Could you check a few things on this model? Use its own coordinates, in mm. Round coordinates to 2 decimals unless told otherwise and drop trailing zeros. Write each loop counter-clockwise with the first axis right and the second up, starting at its lowest first coordinate (ties: lowest second). Pieces come first, ordered by that corner, then holes. Notation, with made-up numbers: M 82,-39.5 L 115,-39.5 A15 ccw 115,-27.5 Z; hole C -25.5,0.5 d4. An arc over 180 degrees is marked long. One line per item, written item: value. Start each with the question number.
(1) I want a section at C-C on x = -9.5. Please give me the cut outline in (y, z).
(2) If I drill on L1, parallel to X at y = -14, z = 1.75; L2, parallel to Y at x = -26, z = 0.5; L3, parallel to X at y = -26, z = 0.5, over which ranges is the centre line in solid material (lowest first)?
(3) I'm going to push a flat-ended pin straight in: pin 1 Ø2.5 at (x, y) = (-36.84, 14.81) entering from +Z. Where does the tip first touch, or does it pass through?
(4) Thinking about a two-plate mould opening in Y: for faces 1 (the face through (39.301, 0, 4)), 2 (the face through (11.99, -24, 3.94)), 3 (the face through (0, -39.298, 4)), which applies, released by +Y, released by -Y, zero draft, split by the parting line, or undercut?
(5) I want a section at B-B on z = 4.75. Count the separate pieces of the cut face and the enclosed holes in it, and give its area (3 significant figures).
(6) I want a section at A-A on x = 7. Please give me the cut outline in (y, z), and give its area (3 significant figures).
```python
from build123d import *

# Parameters (mm, degrees)
SKETCH1_W           = 78.25
SKETCH1_H           = 79.3
SKETCH1_R           = 5
SKETCH1_R_2         = 2
SKETCH1_R_3         = 1.5
BOSS_EXTRUDE1_DEPTH = 8


with BuildPart() as part:
    # Sketch1 → Boss-Extrude1 (new body)
    with BuildSketch(Plane.XY):
        with Locations((0.176122561, 0.352245122)):
            Rectangle(SKETCH1_W, SKETCH1_H)
        with Locations((-9.875194839, -28.39441243)):
            Circle(SKETCH1_R, mode=Mode.SUBTRACT)
        with Locations((9.301122561, -28.217424669)):
            Circle(SKETCH1_R, mode=Mode.SUBTRACT)
        with Locations(Location((-28.948877439, -28.303646558, 0), (0, 0, 180))):
            Circle(SKETCH1_R, mode=Mode.SUBTRACT)
        with Locations((-26.677304512, 19.502245122)):
            Circle(SKETCH1_R_2, mode=Mode.SUBTRACT)
        with Locations((-26.677304512, -8.437754878)):
            Circle(SKETCH1_R_2, mode=Mode.SUBTRACT)
        with Locations((24.122695488, -23.677754878)):
            Circle(SKETCH1_R_2, mode=Mode.SUBTRACT)
        with Locations((25.392695488, 24.582245122)):
            Circle(SKETCH1_R_2, mode=Mode.SUBTRACT)
        with Locations((-36.837723202, 14.814078865)):
            Circle(SKETCH1_R_3, mode=Mode.SUBTRACT)
        with Locations((-36.837723202, -14.185921135)):
            Circle(SKETCH1_R_3, mode=Mode.SUBTRACT)
        with Locations((37.162276798, -14.185921135)):
            Circle(SKETCH1_R_3, mode=Mode.SUBTRACT)
        with Locations((37.162276798, 14.814078865)):
            Circle(SKETCH1_R_3, mode=Mode.SUBTRACT)
    extrude(amount=BOSS_EXTRUDE1_DEPTH)


solid = part.part
```
Found:
1. outline: M -39.3,0 L -33.38,0 L -33.38,8 L -39.3,8 Z; M -23.41,0 L 40,0 L 40,8 L -23.41,8 Z
2. L1: x = -38.95 to -38.33, -35.35 to 35.67, 38.65 to 39.3
2. L2: y = -39.3 to -32.34, -24.27 to -10.32, -6.56 to 17.62, 21.38 to 40
2. L3: x = -38.95 to -33.39, -24.51 to -14.26, -5.49 to 4.82, 13.78 to 39.3
3. pin 1: passes through
4. face 1: zero draft
4. face 2: undercut
4. face 3: released by -Y
5. separate pieces: 1
5. enclosed holes: 11
5. area: 5,890 mm²
6. outline: M -39.3,0 L -32.66,0 L -32.66,8 L -39.3,8 Z; M -23.78,0 L 40,0 L 40,8 L -23.78,8 Z
6. area: 563 mm²
